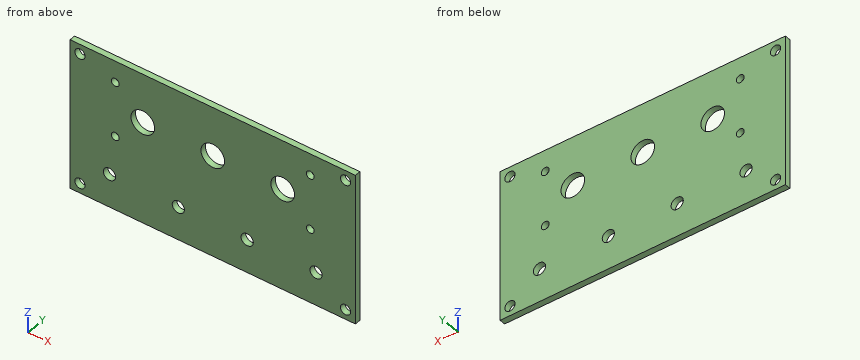
from build123d import *

# Parameters (mm, degrees)
SKETCH1_W           = 145
SKETCH1_H           = 77
SKETCH1_R           = 3.1
SKETCH1_R_2         = 2.6
SKETCH1_R_3         = 6
SKETCH1_R_4         = 2
BOSS_EXTRUDE1_DEPTH = 3


with BuildPart() as part:
    # Sketch1 → Boss-Extrude1 (new body)
    with BuildSketch(Plane(origin=(0, 0, 0), x_dir=(1, 0, 0), z_dir=(0, 1, 0))):
        with Locations((72.5, 38.5)):
            Rectangle(SKETCH1_W, SKETCH1_H)
        with Locations(Location((20, 60, 0), (0, 0, 270))):
            Circle(SKETCH1_R, mode=Mode.SUBTRACT)
        with Locations(Location((55, 60, 0), (0, 0, 270))):
            Circle(SKETCH1_R, mode=Mode.SUBTRACT)
        with Locations(Location((90, 60, 0), (0, 0, 270))):
            Circle(SKETCH1_R, mode=Mode.SUBTRACT)
        with Locations(Location((125, 60, 0), (0, 0, 270))):
            Circle(SKETCH1_R, mode=Mode.SUBTRACT)
        with Locations(Location((5, 72, 0), (0, 0, 270))):
            Circle(SKETCH1_R_2, mode=Mode.SUBTRACT)
        with Locations(Location((5, 5, 0), (0, 0, 270))):
            Circle(SKETCH1_R_2, mode=Mode.SUBTRACT)
        with Locations(Location((140, 5, 0), (0, 0, 270))):
            Circle(SKETCH1_R_2, mode=Mode.SUBTRACT)
        with Locations(Location((140, 72, 0), (0, 0, 270))):
            Circle(SKETCH1_R_2, mode=Mode.SUBTRACT)
        with Locations(Location((36.94, 25, 0), (0, 0, 270))):
            Circle(SKETCH1_R_3, mode=Mode.SUBTRACT)
        with Locations(Location((72.5, 25, 0), (0, 0, 270))):
            Circle(SKETCH1_R_3, mode=Mode.SUBTRACT)
        with Locations(Location((108.06, 25, 0), (0, 0, 270))):
            Circle(SKETCH1_R_3, mode=Mode.SUBTRACT)
        with Locations(Location((22.94, 39, 0), (0, 0, 270))):
            Circle(SKETCH1_R_4, mode=Mode.SUBTRACT)
        with Locations(Location((122.06, 39, 0), (0, 0, 270))):
            Circle(SKETCH1_R_4, mode=Mode.SUBTRACT)
        with Locations(Location((122.06, 11, 0), (0, 0, 270))):
            Circle(SKETCH1_R_4, mode=Mode.SUBTRACT)
        with Locations(Location((22.94, 11, 0), (0, 0, 270))):
            Circle(SKETCH1_R_4, mode=Mode.SUBTRACT)
    extrude(amount=BOSS_EXTRUDE1_DEPTH)


solid = part.part
The model under review builds one solid part; all positions refer to its coordinate system, in mm. Give positions to 0.01 mm unless a question says otherwise; leave off trailing zeros. Order: outer loops, then holes, each group sorted by start corner. A loop starts at its lowest first (then second) coordinate and runs counter-clockwise, first axis right, second up. Notation, with made-up numbers: M -4.5,-36 L 3.5,-36 A19 cw 3.5,-17 Z; hole C 78,-34.75 d2. An arc over 180 degrees is marked long. Answer in a Markdown table with one row per item. Add a question column.
1. For pin 1 Ø8.5 at (x, z) = (5, -5) entering from -Y, flat-tipped, find the tip position at first contact; note if it passes through.
2. Add section A-A on x = 72.5. State the section outline as (y, z) points.
3. Add section B-B on z = -60. State the section outline as (x, y) points.
4. Add section D-D on z = -72. State the section outline as (x, y) points, plus the area to 3 significant figures.
5. Add section C-C on y = 1.35. Count the separate pieces of the cut face and the enclosed holes in it, plus the area to 3 significant figures.
6. To check wall thickness, follow line 1 along X through (y, z) = (0.6, -39); line 2 along X through (y, z) = (0.4, -5); line 3 along X through (y, z) = (1.75, -60). State the ranges of each line that lie inside material, in increasing order.
The answers:
| question | item | result |
|---|---|---|
| 1 | pin 1 | y = 0 |
| 2 | outline | M 0,-77 L 3,-77 L 3,-31 L 0,-31 Z; M 0,-19 L 3,-19 L 3,0 L 0,0 Z |
| 3 | outline | M 0,0 L 16.9,0 L 16.9,3 L 0,3 Z; M 23.1,0 L 51.9,0 L 51.9,3 L 23.1,3 Z; M 58.1,0 L 86.9,0 L 86.9,3 L 58.1,3 Z; M 93.1,0 L 121.9,0 L 121.9,3 L 93.1,3 Z; M 128.1,0 L 145,0 L 145,3 L 128.1,3 Z |
| 4 | outline | M 0,0 L 2.4,0 L 2.4,3 L 0,3 Z; M 7.6,0 L 137.4,0 L 137.4,3 L 7.6,3 Z; M 142.6,0 L 145,0 L 145,3 L 142.6,3 Z |
| 4 | area | 404 mm2 |
| 5 | separate pieces | 1 |
| 5 | enclosed holes | 15 |
| 5 | area | 10,600 mm2 |
| 6 | line 1 | 0 to 20.94, 24.94 to 120.06, 124.06 to 145 |
| 6 | line 2 | 0 to 2.4, 7.6 to 137.4, 142.6 to 145 |
| 6 | line 3 | 0 to 16.9, 23.1 to 51.9, 58.1 to 86.9, 93.1 to 121.9, 128.1 to 145 |
